from build123d import *

# Parameters (mm, degrees)
SKETCH2_R          = 3
CUT_EXTRUDE1_DEPTH = 100
CIRPATTERN1_COUNT  = 8
FILLET1_R          = 2


with BuildPart() as part:
    # Sketch1 → Revolve1 (revolve)
    with BuildSketch(Plane(origin=(0, 0, 0), x_dir=(1, 0, 0), z_dir=(0, 1, 0)), mode=Mode.PRIVATE) as revolve1_sk:
        Polygon((0, 0), (0, 26.45), (2, 26.45), (2, 23.45), (6, 23.45), (6, 26.45), (22, 26.45), (22, 22.45), (4, 22.45), (4, 0), align=None)
    revolve(revolve1_sk.sketch.rotate(Axis((0, 0, 0), (1, 0, 0)), 180), axis=Axis((0, 0, 0), (1, 0, 0)))

    # Sketch2 → Cut-Extrude1 (cut)
    with BuildSketch(Plane(origin=(0, 0, 0), x_dir=(1, 0, 0), z_dir=(0, 1, 0))):
        with Locations(Location((14, 0, 0), (0, 0, 270))):
            Circle(SKETCH2_R)
    cut_extrude1 = extrude(amount=-CUT_EXTRUDE1_DEPTH, mode=Mode.SUBTRACT)

    # CirPattern1: Cut-Extrude1 ×8 about axis
    cirpattern1_axis = Axis((4, 0, 0), (1, 0, 0))
    for i in range(1, CIRPATTERN1_COUNT):
        add(cut_extrude1.rotate(cirpattern1_axis, i * 360 / CIRPATTERN1_COUNT), mode=Mode.SUBTRACT)

    # Fillet1
    fillet1_edges = [part.edges().sort_by_distance(p)[0] for p in [
        (4, 0, -22.45),
    ]]
    fillet(fillet1_edges, radius=FILLET1_R)


solid = part.part
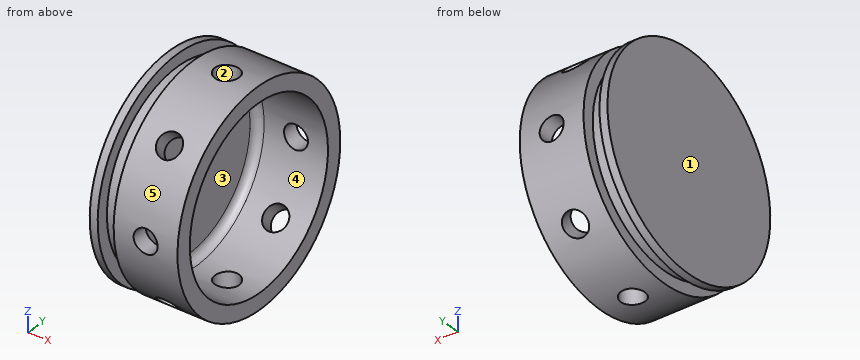
Check sheet for the modelled part. Datum: model origin and axes. Units: mm. Face numbers are marked on the shaded views. A direction names the side the tool comes from. Give positions to 0.01 mm unless a question says otherwise; leave off trailing zeros. Loops run counter-clockwise (first coordinate to the right, second up) from the corner with the lowest first, then second, coordinate; pieces in that order, holes last. Notation, with made-up numbers: M -8.75,-9.75 L 26.25,-9.75 A31 ccw 26.25,22.25 Z; hole C -6,-5 d10. An arc over 180 degrees is marked long. Answer as a JSON object with one key per item and string values. Group by question number.
Q1. Cross-section at D-D on x = 6.75. Record the cut outline in (y, z), then the cut area to 3 significant figures.
Q2. Release check for a two-part mould opening along X. For the marked faces 1, 2 and 3 record: released by +X, released by -X, zero draft, split by the parting line, or undercut.
Q3. Cross-section at C-C on x = 16. Give the number of separate pieces and of enclosed holes in the cut face, then the cut area to 3 significant figures.
Q4. Material ranges on line 1 along X through (y, z) = (-23.8, 0); line 2 along X through (y, z) = (11, -23); line 3 along Z through (x, y) = (14.25, 5), recorded low to high. Write a range as [from, to].
Q5. Cross-section at A-A on y = 0. Record the cut outline in (x, z).
Q6. Access from +Z, -Z, +X, -X, +Y, -Y to the whole of each face (thin tool, end or side, straight path). Record for the marked faces 4 and 5.
Q7. Go/stop test with flat-tipped pins: P1, Ø2, axis at x = 12.5, y = -16, coming from the -Z side; P2, Ø1, axis at x = 18.5, z = -14, coming from the -Y side; P3, Ø2, axis at y = -5.5, z = -16.5, coming from the +X side. Record where each tip stops, or that it passes through.
Evaluation:
{
 "1": {"outline": "C 0,0 d52.9; hole C 0,0 d44.9", "area": "614 mm2"},
 "2": {"face 1": "released by -X", "face 2": "undercut", "face 3": "released by +X"},
 "3": {"separate pieces": "8", "enclosed holes": "0", "area": "471 mm2"},
 "4": {"line 1": "x = [0, 2], [6, 11], [17, 22]", "line 2": "x = [0, 2], [6, 22]", "line 3": "z = [-25.97, -21.89], [21.89, 25.97]"},
 "5": {"outline": "M 0,-26.45 L 2,-26.45 L 2,-23.45 L 6,-23.45 L 6,-26.45 L 11,-26.45 L 11,-22.45 L 6,-22.45 A2 cw 4,-20.45 L 4,20.45 A2 cw 6,22.45 L 11,22.45 L 11,26.45 L 6,26.45 L 6,23.45 L 2,23.45 L 2,26.45 L 0,26.45 Z; M 17,-26.45 L 22,-26.45 L 22,-22.45 L 17,-22.45 Z; M 17,22.45 L 22,22.45 L 22,26.45 L 17,26.45 Z"},
 "6": {"face 4": "+X", "face 5": "+X, -X"},
 "7": {"P1": "stops at z = -21.79", "P2": "stops at y = -22.75", "P3": "stops at x = 4"}
}
